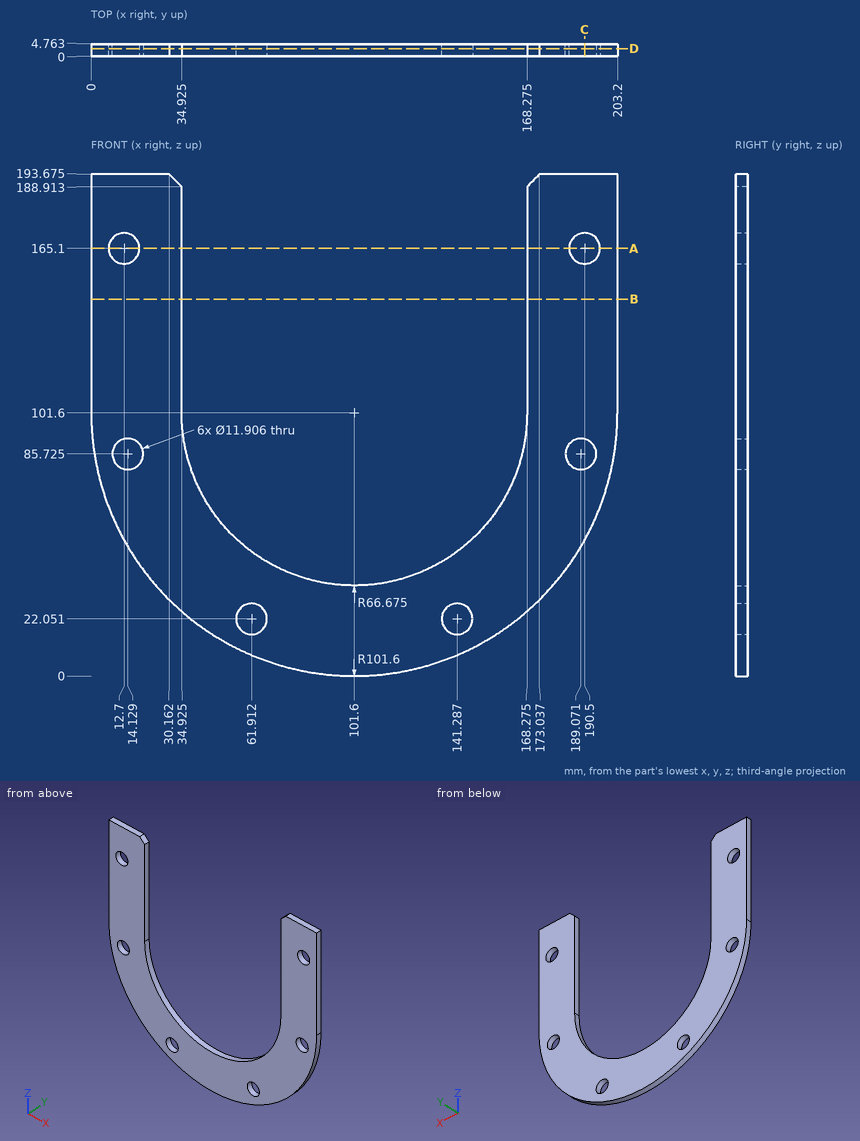
Could you check a few things on this drawing? It's one solid part, dimensions in mm from its lowest x, y, z. Give positions to 0.01 mm unless a question says otherwise; leave off trailing zeros. Loops run counter-clockwise (first coordinate to the right, second up) from the corner with the lowest first, then second, coordinate; pieces in that order, holes last. Notation, with made-up numbers: (-27.5, -25.5) -> (7.5, -25.5) arc R21 ccw to (7.5, -4.5) -> close; hole circle Ø7 at (-19, 18). An arc over 180 degrees is marked (long way). Use one line per item in the form item = value. Start each with the question number.
1) Imagine slicing it at A-A (z = 165.1). Please give me the cut outline in (x, y) (1 decimal).
2) Please list where these lines run through material, in increasing order: line 1 along X through (y, z) = (3.25, 103) (1 decimal); line 2 along X through (y, z) = (3.2, 169) (1 decimal); line 3 along X through (y, z) = (0.8, 169.5) (1 decimal).
3) Imagine slicing it at B-B (z = 145.5). Please give me the cut outline in (x, y) (1 decimal).
4) Imagine slicing it at D-D (y = 2.95). Count the separate pieces of the cut face and the enclosed holes in it, then the cut area to 3 significant figures.
5) Imagine slicing it at C-C (x = 190.5). Please give me the cut outline in (y, z) (1 decimal).
Check values:
q1.outline = (0, 0) -> (6.7, 0) -> (6.7, 4.8) -> (0, 4.8) -> close; (18.7, 0) -> (34.9, 0) -> (34.9, 4.8) -> (18.7, 4.8) -> close; (168.3, 0) -> (184.5, 0) -> (184.5, 4.8) -> (168.3, 4.8) -> close; (196.5, 0) -> (203.2, 0) -> (203.2, 4.8) -> (196.5, 4.8) -> close
q2.line_1 = 0 to 34.9, 168.3 to 203.2
q2.line_2 = 0 to 8.2, 17.2 to 34.9, 168.3 to 186, 195 to 203.2
q2.line_3 = 0 to 8.7, 16.7 to 34.9, 168.3 to 186.5, 194.5 to 203.2
q3.outline = (0, 0) -> (34.9, 0) -> (34.9, 4.8) -> (0, 4.8) -> close; (168.3, 0) -> (203.2, 0) -> (203.2, 4.8) -> (168.3, 4.8) -> close
q4.separate_pieces = 1
q4.enclosed_holes = 6
q4.area = 15,000 mm^2
q5.outline = (0, 52.4) -> (4.8, 52.4) -> (4.8, 79.9) -> (0, 79.9) -> close; (0, 91.5) -> (4.8, 91.5) -> (4.8, 159.1) -> (0, 159.1) -> close; (0, 171.1) -> (4.8, 171.1) -> (4.8, 193.7) -> (0, 193.7) -> close
